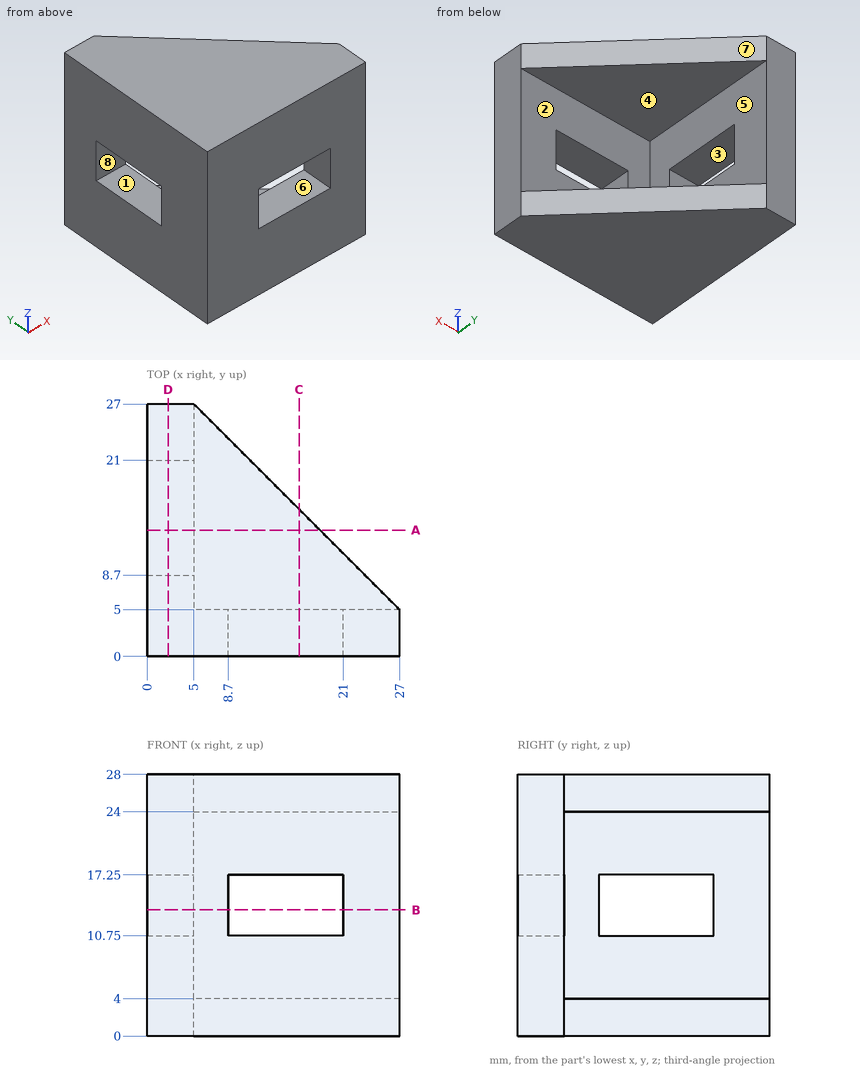
Here's the drawing with two shaded views (mm, measured from the low corner). I have some questions. A direction names the side the tool comes from. Round coordinates to 2 decimals unless told otherwise and drop trailing zeros. Write each loop counter-clockwise with the first axis right and the second up, starting at its lowest first coordinate (ties: lowest second). Pieces come first, ordered by that corner, then holes. Notation, with made-up numbers: M 19.25,-40 L 43.25,-40 A17 ccw 43.25,-28 Z; hole C -22,29 d9. An arc over 180 degrees is marked long. Write each question's results on one line, items separated by ' | '. Start each with the question number.
1. Imagine slicing it at B-B on z = 13.5. List the corners of the cut face in (x, y) for me.
2. Imagine slicing it at A-A on y = 13.5. List the corners of the cut face in (x, z) for me.
3. On a 3-axis mill with a long thin cutter (end or side, diameter ignored), from which of +Z, -Z, +X, -X, +Y, -Y can I reach the whole of each face in a straight line? I mean the marked faces 5, 6, 7 and 8. Say none if no direction works.
4. I need wall thicknesses on L1, parallel to Z at x = 10.25, y = 9.25; L2, parallel to Y at x = 17, z = 20. Which ranges of each line are inside material? Lowest first, please. Write a range as from..to.
5. Imagine slicing it at D-D on x = 2.25. List the corners of the cut face in (y, z) for me.
6. I'm going to push flat-ended pins straight in: pin 1 Ø6 at (y, z) = (17.5, 12) entering from +X; pin 2 Ø6 at (x, z) = (15.5, 10.5) entering from +Y. Where does each tip first touch, or does it pass through?
7. Thinking about a two-plate mould opening in Y: for the marked faces 1, 2, 3 and 4, which applies, +Y half, -Y half, draft (parallel to the pull), parting line (faces both ways), or undercut?
8. Imagine slicing it at C-C on x = 16.25. List the corners of the cut face in (y, z) for me.
Result sheet:
1) outline: M 0,0 L 8.7,0 L 8.7,5 L 5,5 L 5,8.7 L 0,8.7 Z; M 0,21 L 5,21 L 5,27 L 0,27 Z; M 21,0 L 27,0 L 27,5 L 21,5 Z
2) outline: M 0,0 L 18.5,0 L 18.5,4 L 5,4 L 5,10.75 L 0,10.75 Z; M 0,17.25 L 5,17.25 L 5,24 L 18.5,24 L 18.5,28 L 0,28 Z
3) face 5: +X, +Y | face 6: +Y, -Y | face 7: +Z, -Z, +X, +Y | face 8: +X, -X
4) L1: z = 0..4, 24..28 | L2: y = 0..5
5) outline: M 0,0 L 27,0 L 27,28 L 0,28 Z; hole M 8.7,10.75 L 21,10.75 L 21,17.25 L 8.7,17.25 Z
6) pin 1: stops at x = 5 | pin 2: stops at y = 5
7) face 1: undercut | face 2: +Y half | face 3: undercut | face 4: draft
8) outline: M 0,0 L 15.75,0 L 15.75,4 L 5,4 L 5,10.75 L 0,10.75 Z; M 0,17.25 L 5,17.25 L 5,24 L 15.75,24 L 15.75,28 L 0,28 Z
